Geometry check sheet. Reference: drawing and pictorial views, mm from the part's lowest x, y, z. Coordinates: 2 decimals unless noted, no trailing zeros. Loops run counter-clockwise (first coordinate to the right, second up) from the corner with the lowest first, then second, coordinate; pieces in that order, holes last. Notation, with made-up numbers: (35.25, 23.5) -> (75.25, 23.5) arc R21 ccw to (75.25, 27.5) -> close; hole circle Ø4 at (4.5, -27.75). An arc over 180 degrees is marked (long way). Answer as a JSON object with one key per item and string values.
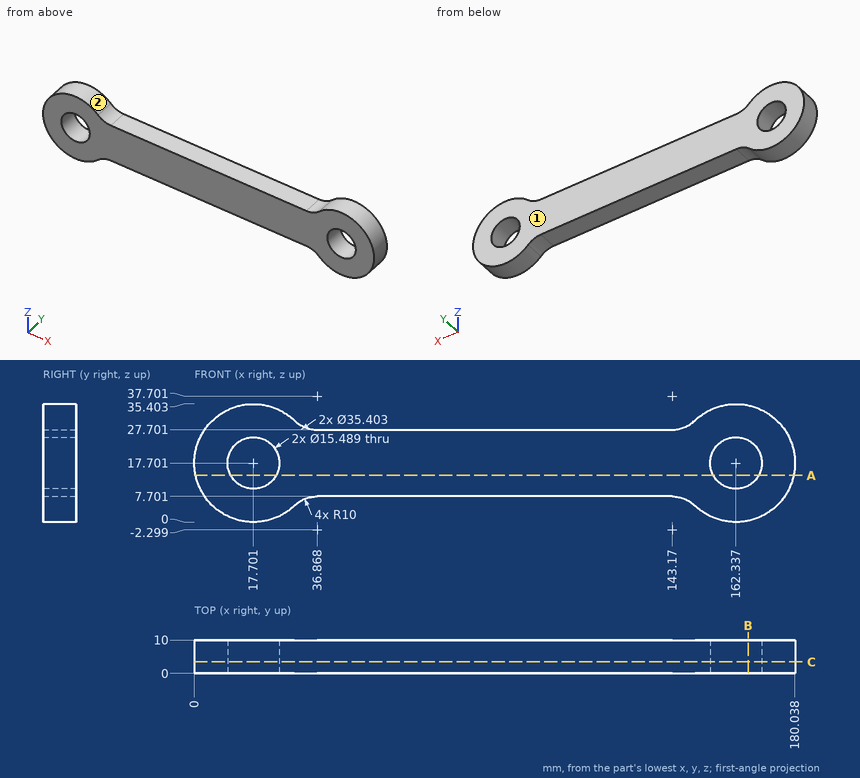
1. Section check B-B, the plane x = 166. Record the boundary of the cut face in (y, z) (1 decimal).
Evaluation:
{"outline": "(0, 0.4) -> (10, 0.4) -> (10, 10.9) -> (0, 10.9) -> close; (0, 24.5) -> (10, 24.5) -> (10, 35) -> (0, 35) -> close"}
2. Depth check by flat-ended pin: P1, Ø18, axis at x = 162.34, z = 17.7, coming from the +Y side; P2, Ø5, axis at x = 130.5, y = 3.5, coming from the -Z side; P3, Ø6, axis at y = 5, z = 29, coming from the -X side (1 decimal); P4, Ø5, axis at y = 3, z = 15, coming from the -X side. Enter the tip coordinate at first touch or a pass-through.
Evaluation:
{"P1": "stops at y = 10", "P2": "stops at z = 7.7", "P3": "stops at x = 2.1", "P4": "stops at x = 0"}
3. Section check A-A, the plane z = 14. Record the boundary of the cut face in (x, y) (1 decimal).
Evaluation:
{"outline": "(0.4, 0) -> (10.9, 0) -> (10.9, 10) -> (0.4, 10) -> close; (24.5, 0) -> (155.5, 0) -> (155.5, 10) -> (24.5, 10) -> close; (169.1, 0) -> (179.6, 0) -> (179.6, 10) -> (169.1, 10) -> close"}
4. Section check C-C, the plane y = 3.5. State how many separate pieces and enclosed holes the cut face has, then the cut area to 3 significant figures.
Evaluation:
{"separate pieces": "1", "enclosed holes": "2", "area": "3,830 mm^2"}
5. Mould release check, pull along X, two halves, no side actions. Record for the marked faces 1 and 2: released by +X, released by -X, zero draft, split by the parting line, or undercut.
Evaluation:
{"face 1": "zero draft", "face 2": "undercut"}
6. Thickness scan on probe 1 along X at (y, z) = (5.75, 11.5) (1 decimal); probe 2 along X at (y, z) = (9, 15.5) (1 decimal); probe 3 along X at (y, z) = (2.5, 5) (1 decimal). Record the ranges inside material, lowest first. Write a range as from..to.
Evaluation:
{"probe 1": "x = 1.1..13.1, 22.3..157.7, 167..178.9", "probe 2": "x = 0.1..10.3, 25.1..154.9, 169.8..179.9", "probe 3": "x = 5.4..30, 150..174.7"}
